For this review, take the finished solid that the model builds, in its own axes (mm). A direction names the side the tool comes from. Round coordinates to 2 decimals unless told otherwise and drop trailing zeros. Order: outer loops, then holes, each group sorted by start corner. A loop starts at its lowest first (then second) coordinate and runs counter-clockwise, first axis right, second up. Notation, with made-up numbers: (52, 0.5) -> (66, 0.5) arc R21 cw to (66, 31.5) -> close; hole circle Ø6 at (25, 5). An arc over 180 degrees is marked (long way). Use a Markdown table: item, result. Add a question column.
1) Consider section B-B (x = 20.5). State the section outline as (y, z) points, plus the area to 3 significant figures.
2) Wall thickness on line 1 along X through (y, z) = (5.25, 4); line 2 along X through (y, z) = (47, 2.5); line 3 along Z through (x, y) = (-20.5, 3.25): over which ranges is each line inside the solid? List them lowest first. Write a range as [from, to].
3) Clearance check with flat-ended pins moving along their axes: P1, Ø2, axis at x = -11, z = 5, coming from the -Y side; P2, Ø2, axis at y = 9.5, z = 7, coming from the +X side; P3, Ø1.5, axis at x = -19.5, z = 1.5, coming from the +Y side; P4, Ø3, axis at y = 49, z = 2, coming from the -X side. State where each tip first meets the part, or that it passes through.
4) Machinability: for faces 5 (the face through (0, 0, 4)), 6 (the face through (-11, 51, 4)), 7 (the face through (-20.5, 8, 0.5)), which of the approach directions +Z, -Z, +X, -X, +Y, -Y give a long, thin tool a straight path to every point of the face, cutting with its end or side? Answer none if there is none.
5) Consider section C-C (y = 14.5). State the section outline as (x, z) points.
6) Consider section A-A (z = 4). State the section outline as (x, y) points, plus the area to 3 significant figures.
7) Draft analysis for pull direction Y (two halves, no side actions). For faces 1 (the face through (20.5, 8, 7.5)), 2 (the face through (7.2, 48, 4)), 3 (the face through (-14.2, 48, 4)), 4 (the face through (-17.5, 31, 4)), state which applies: pulls with the +Y half, pulls with the -Y half, needs draft (parallel to the pull), parting line crosses it, or undercut.
```python
from build123d import *

# Parameters (mm, degrees)
SKETCH2_W                                      = 7
SKETCH2_H                                      = 6
BOSS_EXTRUDE1_DEPTH                            = 8
CSK_FOR_M3_FLAT_HEAD_MACHINE_SCREW1_AT_2_COUNT = 2
CSK_FOR_M3_FLAT_HEAD_MACHINE_SCREW1_AT_2_PITCH = 41


with BuildPart() as part:
    # Sketch2 → Boss-Extrude1 (new body)
    with BuildSketch(Plane.XY):
        Polygon((23.5, 0), (-23.5, 0), (-23.5, 8), (-17.5, 8), (-17.5, 55), (17.5, 55), (17.5, 8), (23.5, 8), align=None)
        with Locations((10.7, 48)):
            Rectangle(SKETCH2_W, SKETCH2_H, mode=Mode.SUBTRACT)
        with Locations((-10.7, 48)):
            Rectangle(SKETCH2_W, SKETCH2_H, mode=Mode.SUBTRACT)
    extrude(amount=BOSS_EXTRUDE1_DEPTH)

    # Sketch4 → CSK for M3 Flat Head Machine Screw1 (revolve, cut)
    with BuildSketch(Plane(origin=(-20.5, 8, 4), x_dir=(0, 0, 1), z_dir=(1, 0, 0))):
        Polygon((0, 0), (0, 8), (1.7, 8), (1.7, 1.45), (3.15, 0), align=None)
    csk_for_m3_flat_head_machine_screw1 = revolve(axis=Axis((-20.5, 14.35, 4), (0, -1, 0)), mode=Mode.SUBTRACT)

    # CSK for M3 Flat Head Machine Screw1 at 2: CSK for M3 Flat Head Machine Screw1 ×2
    with Locations(*[(i * CSK_FOR_M3_FLAT_HEAD_MACHINE_SCREW1_AT_2_PITCH, 0, 0) for i in range(1, CSK_FOR_M3_FLAT_HEAD_MACHINE_SCREW1_AT_2_COUNT)]):
        add(csk_for_m3_flat_head_machine_screw1, mode=Mode.SUBTRACT)


solid = part.part
```
Results list:
| question | item | result |
|---|---|---|
| 1 | outline | (0, 0) -> (8, 0) -> (8, 0.85) -> (6.55, 2.3) -> (0, 2.3) -> close; (0, 5.7) -> (6.55, 5.7) -> (8, 7.15) -> (8, 8) -> (0, 8) -> close |
| 1 | area | 34.7 mm2 |
| 2 | line 1 | [-23.5, -22.2], [-18.8, 18.8], [22.2, 23.5] |
| 2 | line 2 | [-17.5, -14.2], [-7.2, 7.2], [14.2, 17.5] |
| 2 | line 3 | [0, 2.3], [5.7, 8] |
| 3 | P1 | y = 0 |
| 3 | P2 | x = 17.5 |
| 3 | P3 | y = 8 |
| 3 | P4 | x = -17.5 |
| 4 | face 5 | +Z, -Z, +X, -X, -Y |
| 4 | face 6 | +Z, -Z |
| 4 | face 7 | +Z, -Z, -X, +Y |
| 5 | outline | (-17.5, 0) -> (17.5, 0) -> (17.5, 8) -> (-17.5, 8) -> close |
| 6 | outline | (-23.5, 0) -> (-22.2, 0) -> (-22.2, 6.55) -> (-23.5, 7.85) -> close; (-18.8, 0) -> (18.8, 0) -> (18.8, 6.55) -> (17.35, 8) -> (17.5, 8) -> (17.5, 55) -> (-17.5, 55) -> (-17.5, 8) -> (-17.35, 8) -> (-18.8, 6.55) -> close; (22.2, 0) -> (23.5, 0) -> (23.5, 7.85) -> (22.2, 6.55) -> close; hole (-14.2, 45) -> (-7.2, 45) -> (-7.2, 51) -> (-14.2, 51) -> close; hole (7.2, 45) -> (14.2, 45) -> (14.2, 51) -> (7.2, 51) -> close |
| 6 | area | 1,880 mm2 |
| 7 | face 1 | pulls with the +Y half |
| 7 | face 2 | undercut |
| 7 | face 3 | undercut |
| 7 | face 4 | needs draft |
